```python
from build123d import *

# Parameters (mm, degrees)
SKETCH1_R           = 3.175
BOSS_EXTRUDE1_DEPTH = 14
CUT_EXTRUDE2_START  = -6.35
CUT_EXTRUDE2_DEPTH  = 6.35
SKETCH7_R           = 3.175
CUT_EXTRUDE4_DEPTH  = 3.05
SKETCH9_R           = 5
SKETCH9_R_2         = 1.3890625
BOSS_EXTRUDE2_DEPTH = 4.6
SKETCH9_3_R         = 1.3890625
CUT_EXTRUDE5_DEPTH  = 4.6


with BuildPart() as part:
    # Sketch1 → Boss-Extrude1 (new body)
    with BuildSketch(Plane.XY):
        Circle(SKETCH1_R)
    extrude(amount=BOSS_EXTRUDE1_DEPTH)

    # Sketch2 → Cut-Extrude2 (cut)
    with BuildSketch(Plane.XY.offset(14).offset(CUT_EXTRUDE2_START)):
        with BuildLine():
            Line((-1.905, 2.54), (-1.905, -2.54))
            ThreePointArc((-1.905, -2.54), (-3.175, 0), (-1.905, 2.54))
        make_face()
    extrude(amount=CUT_EXTRUDE2_DEPTH, mode=Mode.SUBTRACT)

    # Sketch7 → Cut-Extrude4 (cut)
    with BuildSketch(Plane(origin=(0, 0, 0), x_dir=(-1, 0, 0), z_dir=(0, 0, -1))):
        with Locations(Location((0, 0, 0), (0, 0, 306.869897646))):
            Circle(SKETCH7_R)
    extrude(amount=-CUT_EXTRUDE4_DEPTH, mode=Mode.SUBTRACT)

    # Sketch9 → Boss-Extrude2 (add)
    with BuildSketch(Plane(origin=(0, 0, 3.05), x_dir=(-1, 0, 0), z_dir=(0, 0, -1))):
        Circle(SKETCH9_R)
        Circle(SKETCH9_R_2, mode=Mode.SUBTRACT)
    extrude(amount=-BOSS_EXTRUDE2_DEPTH)

    # Sketch9<3> → Cut-Extrude5 (cut)
    with BuildSketch(Plane(origin=(0, 0, 3.05), x_dir=(-1, 0, 0), z_dir=(0, 0, -1))):
        Circle(SKETCH9_3_R)
    extrude(amount=-CUT_EXTRUDE5_DEPTH, mode=Mode.SUBTRACT)


solid = part.part
```
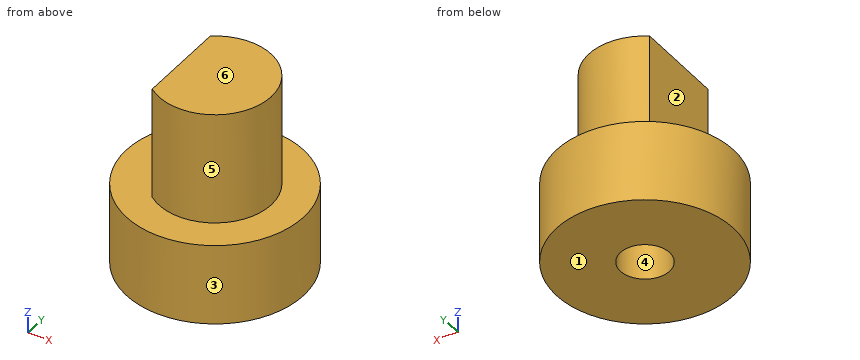
Here's how the part is built. I have some questions about the finished solid (model axes, mm). Face numbers are marked on the shaded views. A direction names the side the tool comes from. Coordinates: 2 decimals unless noted, no trailing zeros. Loops run counter-clockwise (first coordinate to the right, second up) from the corner with the lowest first, then second, coordinate; pieces in that order, holes last. Notation, with made-up numbers: (72, 38.5) -> (97, 38.5) arc R6 cw to (97, 49.5) -> close; hole circle Ø3 at (56.5, 82.5). An arc over 180 degrees is marked (long way). Return JSON: item names as keys, results as strings.
1) Will these pins go through, and if not, where does the flat tip stop? pin 1 (2.5 mm diameter, centred on y = 0.5, z = 11, fed in from -X) (3 decimals); pin 2 (1.5 mm diameter, centred on y = -4, z = 5.5, fed in from -X); pin 3 (1 mm diameter, centred on x = 2.5, z = 4.5, fed in from -Y).
Results below:
{"pin 1": "x = -1.905", "pin 2": "x = -3.8", "pin 3": "y = -4.58"}
2) If we section it at D-D, the plane y = -2.75: Write out the boundary of the cut face in (x, z).
Results below:
{"outline": "(-4.18, 3.05) -> (4.18, 3.05) -> (4.18, 7.65) -> (1.59, 7.65) -> (1.59, 14) -> (-1.59, 14) -> (-1.59, 7.65) -> (-4.18, 7.65) -> close"}
3) If we section it at C-C, the plane z = 8.25: Write out the boundary of the cut face in (x, y) (3 decimals).
Results below:
{"outline": "(-1.905, -2.54) arc R3.175 ccw (long way) to (-1.905, 2.54) -> close"}
4) If we section it at B-B, the plane x = 0: Write out the boundary of the cut face in (y, z) (3 decimals).
Results below:
{"outline": "(-5, 3.05) -> (-1.389, 3.05) -> (-1.389, 7.65) -> (1.389, 7.65) -> (1.389, 3.05) -> (5, 3.05) -> (5, 7.65) -> (3.175, 7.65) -> (3.175, 14) -> (-3.175, 14) -> (-3.175, 7.65) -> (-5, 7.65) -> close"}
5) I need wall thicknesses on line 1 (Y direction, x = 0, z = 4.9); line 2 (Z direction, x = -4.25, y = -0.5); line 3 (X direction, y = -0.5, z = 3.75). Which ranges of each line are inside material? Lowest first, please. Write a range as from..to.
Results below:
{"line 1": "-5..-1.39, 1.39..5", "line 2": "3.05..7.65", "line 3": "-4.97..-1.3, 1.3..4.97"}
6) Thinking about a two-plate mould opening in X: for the marked faces 1, 2, 3 and 4, which applies, +X half, -X half, draft (parallel to the pull), parting line (faces both ways), or undercut?
Results below:
{"face 1": "draft", "face 2": "-X half", "face 3": "parting line", "face 4": "undercut"}
7) If we section it at A-A, the plane y = 0: Write out the boundary of the cut face in (x, z) (3 decimals).
Results below:
{"outline": "(-5, 3.05) -> (-1.389, 3.05) -> (-1.389, 7.65) -> (1.389, 7.65) -> (1.389, 3.05) -> (5, 3.05) -> (5, 7.65) -> (3.175, 7.65) -> (3.175, 14) -> (-1.905, 14) -> (-1.905, 7.65) -> (-5, 7.65) -> close"}
8) For the marked faces 5 and 6, which set-ups out of +Z, -Z, +X, -X, +Y, -Y let a thin tool reach every point of the face, with its end or its side?
Results below:
{"face 5": "+Z", "face 6": "+Z, +X, -X, +Y, -Y"}
